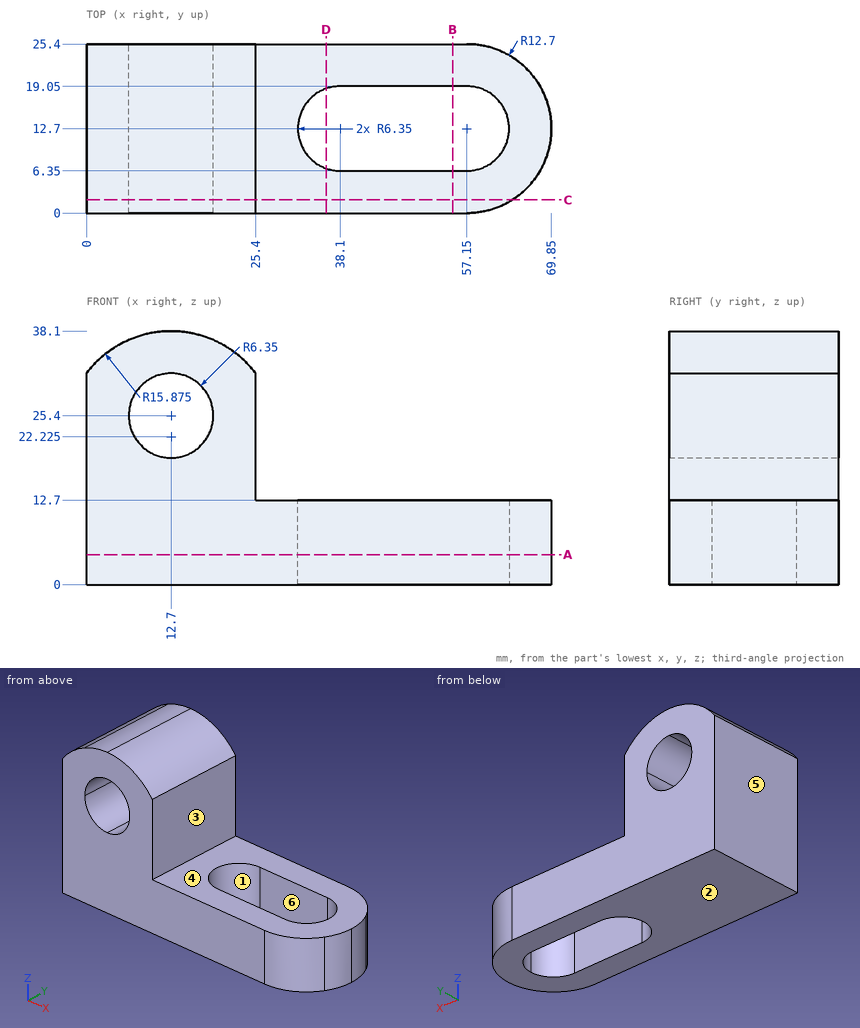
Study the drawing (mm; zero at the part's minimum x, y, z) and answer. A direction names the side the tool comes from. Round coordinates to 2 decimals unless told otherwise and drop trailing zeros. Write each loop counter-clockwise with the first axis right and the second up, starting at its lowest first coordinate (ties: lowest second). Pieces come first, ordered by that corner, then holes.
1) Flat-ended cylindrical pins translate along their axes: P1, Ø8, axis at y = 18.5, z = 33.5, coming from the +X side; P2, Ø6, axis at x = 33, y = 19, coming from the +Z side. Find the tip coordinate at first contact, or state that the pin passes through.
2) Determine the mould class of the marked faces 1, 2 and 3 for opening direction X: pulls with the +X half, pulls with the -X half, needs draft (parallel to the pull), parting line crosses it, or undercut.
3) Which of the six approach directions +Z, -Z, +X, -X, +Y, -Y give full straight-line access (tool end or side, diameter ignored) to the marked faces 4, 5 and 6?
4) A cutting plane is placed at C-C on y = 2. Determine the outline of the cut face in (x, z) (3 decimals).
5) A cutting plane is placed at B-B on x = 55. Determine the outline of the cut face in (y, z), and give its area (3 significant figures).
6) A cutting plane is placed at D-D on x = 36. Determine the outline of the cut face in (y, z).
7) Consider probe 1 along Y at (x, z) = (38.5, 8); probe 2 along Z at (x, y) = (12.5, 7.5); probe 3 along Z at (x, y) = (32, 21.75). Determine where each line is inside the solid, lowest interval first.
8) A cutting plane is placed at A-A on z = 4.5. Determine the outline of the cut face in (x, y).
Entries:
1. P1: stops at x = 25.4
1. P2: stops at z = 12.7
2. face 1: undercut
2. face 2: needs draft
2. face 3: pulls with the +X half
3. face 4: +Z, +X, +Y, -Y
3. face 5: +Z, -Z, -X, +Y, -Y
3. face 6: +Z, -Z
4. outline: (0, 0) - (63.991, 0) - (63.991, 12.7) - (25.4, 12.7) - (25.4, 31.75) arc R15.875 ccw to (0, 31.75) - close; hole circle Ø12.7 at (12.7, 25.4)
5. outline: (0, 0) - (6.35, 0) - (6.35, 12.7) - (0, 12.7) - close; (19.05, 0) - (25.4, 0) - (25.4, 12.7) - (19.05, 12.7) - close
5. area: 161 mm2
6. outline: (0, 0) - (6.71, 0) - (6.71, 12.7) - (0, 12.7) - close; (18.69, 0) - (25.4, 0) - (25.4, 12.7) - (18.69, 12.7) - close
7. probe 1: y = 0 to 6.35, 19.05 to 25.4
7. probe 2: z = 0 to 19.05, 31.75 to 38.1
7. probe 3: z = 0 to 12.7
8. outline: (0, 0) - (57.15, 0) arc R12.7 ccw to (57.15, 25.4) - (0, 25.4) - close; hole (38.1, 6.35) - (57.15, 6.35) arc R6.35 ccw to (57.15, 19.05) - (38.1, 19.05) arc R6.35 ccw to start
